Answer from the drawing. Dimensions are ordinates in mm from the lowest x, y and z of the part. A direction names the side the tool comes from. Give positions to 0.01 mm unless a question says otherwise; leave off trailing zeros. Loops run counter-clockwise (first coordinate to the right, second up) from the corner with the lowest first, then second, coordinate; pieces in that order, holes last. Notation, with made-up numbers: (89.5, 15.5) - (119.5, 15.5) arc R6 ccw to (119.5, 21.5) - close; hole circle Ø7 at (71.25, -4.5). An arc over 180 degrees is marked (long way). Write each question's results on one line, items separated by ' | '. Start each with the question number.
Q1. The part is cut by section C-C, the plane x = 2.5. Write down the section's boundary in (y, z).
Q2. The part is cut by section D-D, the plane x = 6.5. Write down the section's boundary in (y, z) (1 decimal).
Q3. The part is cut by section A-A, the plane y = 10. Write down the section's boundary in (x, z).
Q4. Find the intervals of material crossed by line 1 (Y direction, x = 0.9, z = 4.5); line 2 (Z direction, x = 4.25, y = 5.5); line 3 (Y direction, x = 6.5, z = 4.25) (1 decimal), in increasing order. Write a range as from..to.
Q5. Determine the mould class of the marked faces 1, 2, 3 and 4 for opening direction Z: +Z half, -Z half, draft (parallel to the pull), parting line (faces both ways), or undercut.
Q6. The part is cut by section B-B, the plane z = 4.5. Write down the section's boundary in (x, y) (1 decimal).
Q7. Given pin 1 (3 mm diameter, centred on x = 5, y = 11, fed in from +Z); pin 2 (2 mm diameter, centred on x = 5.5, y = 15, fed in from -Z); pin 3 (2 mm diameter, centred on x = 7, y = 14.5, fed in from +Z), each flat-ended and moving along its own axis, determine where each tip first touches the part or whether it passes through.
Q8. For the marked faces 5 and 6, determine the directions among +Z, -Z, +X, -X, +Y, -Y from which every point of the face is accessible in a straight line to the end or side of a thin tool.
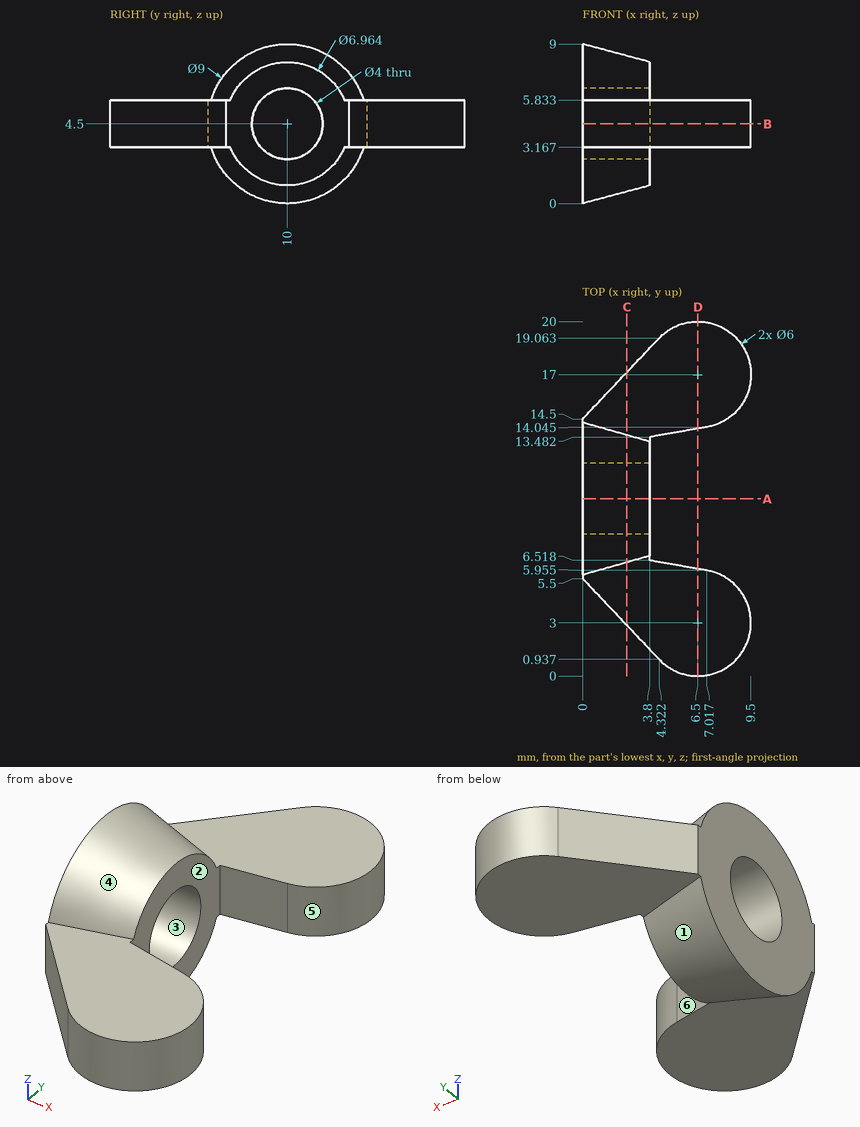
Check sheet entries:
1) outline: (2.86, 3.17) - (6.41, 3.17) arc R3.83 ccw to (13.59, 3.17) - (17.14, 3.17) - (17.14, 5.83) - (13.59, 5.83) arc R3.83 ccw to (6.41, 5.83) - (2.86, 5.83) - close; hole circle Ø4 at (10, 4.5)
2) outline: (0, 3.2) - (6, 3.2) - (6, 5.8) - (0, 5.8) - close; (14, 3.2) - (20, 3.2) - (20, 5.8) - (14, 5.8) - close
3) outline: (0, 0) - (3.8, 1.02) - (3.8, 2.5) - (0, 2.5) - close; (0, 6.5) - (3.8, 6.5) - (3.8, 7.98) - (0, 9) - close
4) line 1: y = 4.55..8, 12..15.45 | line 2: z = 3.17..5.83 | line 3: y = 0..6, 14..20
5) face 1: -Z half | face 2: draft | face 3: undercut | face 4: +Z half
6) outline: (0, 5.5) - (4.3, 0.9) arc R3 ccw (long way) to (7, 6) - (3.8, 6.5) - (3.8, 8) - (0, 8) - close; (0, 12) - (3.8, 12) - (3.8, 13.5) - (7, 14) arc R3 ccw (long way) to (4.3, 19.1) - (0, 14.5) - close
7) pin 1: stops at z = 8.01 | pin 2: stops at z = 3.17 | pin 3: stops at z = 5.83
8) face 5: +Z, -Z | face 6: +Z, -Z, +X
